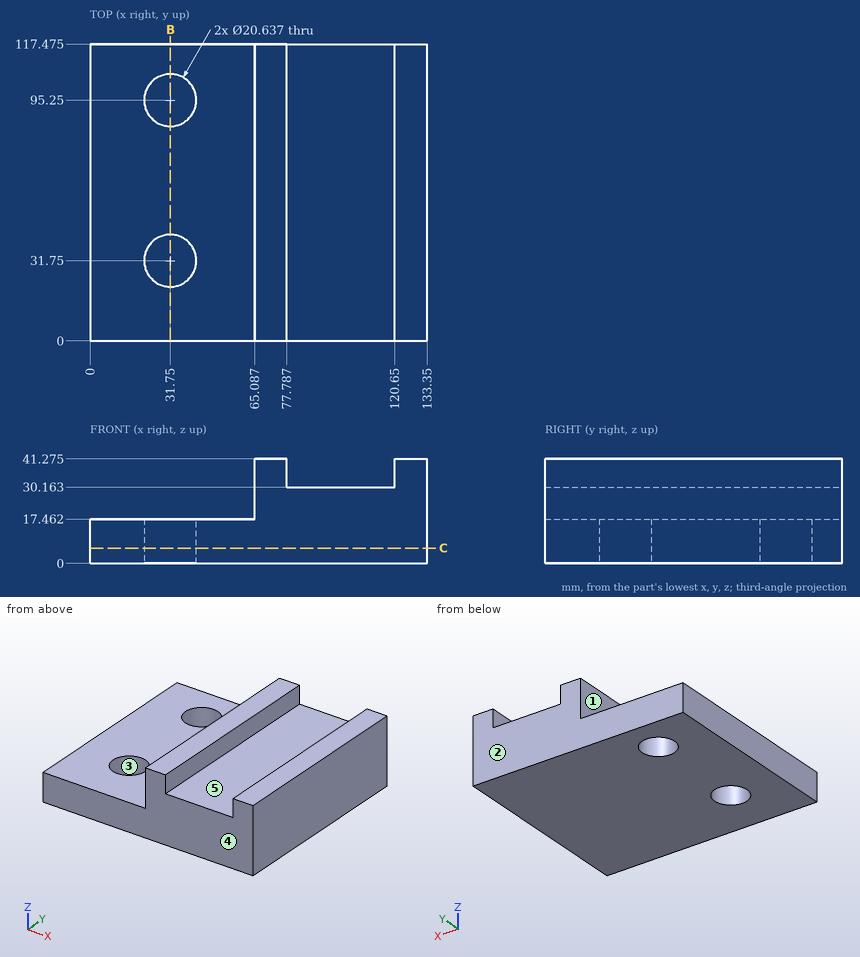
Print and shaded views of the part. All mm, measured from the part's lowest x, y and z. A direction names the side the tool comes from. Coordinates: 2 decimals unless noted, no trailing zeros. Order: outer loops, then holes, each group sorted by start corner. A loop starts at its lowest first (then second) coordinate and runs counter-clockwise, first axis right, second up.
(1) Slice it at B-B, the plane x = 31.75. Write the cut outline in (y, z) (1 decimal).
Check sheet entries:
outline: (0, 0) - (21.4, 0) - (21.4, 17.5) - (0, 17.5) - close; (42.1, 0) - (84.9, 0) - (84.9, 17.5) - (42.1, 17.5) - close; (105.6, 0) - (117.5, 0) - (117.5, 17.5) - (105.6, 17.5) - close
(2) Slice it at C-C, the plane z = 6. State how many separate pieces and enclosed holes the cut face has, and give its area (3 significant figures).
Check sheet entries:
separate pieces: 1
enclosed holes: 2
area: 15,000 mm2
(3) Pull direction Y, two halves, no side cores. Call the marked faces 3, 4 and 5: pulls with the +Y half, pulls with the -Y half, needs draft (parallel to the pull), parting line crosses it, or undercut.
Check sheet entries:
face 3: undercut
face 4: pulls with the -Y half
face 5: needs draft
(4) Tool access for the marked faces 1 and 2: list every direction of +Z, -Z, +X, -X, +Y, -Y with a clear straight run to the whole face (end or side of a thin tool).
Check sheet entries:
face 1: +Z, -X, +Y, -Y
face 2: +Z, -Z, +X, -X, +Y
(5) Probe L1, parallel to Y at x = 31, z = 12 (1 decimal); L2, parallel to Y at x = 31.75, z = 4.5 (1 decimal); L3, parallel to X at y = 58, z = 37. List the from-to ranges inside material, lowest first.
Check sheet entries:
L1: y = 0 to 21.5, 42 to 85, 105.5 to 117.5
L2: y = 0 to 21.4, 42.1 to 84.9, 105.6 to 117.5
L3: x = 65.09 to 77.79, 120.65 to 133.35
(6) Pin check, flat tips, straight feed: pin 1 Ø6 at (y, z) = (21, 30.5) entering from -X; pin 2 Ø16.5 at (x, y) = (31.75, 31.75) entering from -Z. Stop position of each tip, or through.
Check sheet entries:
pin 1: stops at x = 65.09
pin 2: passes through
